Input: dimensioned drawing with shaded views. Units: mm. Origin: part minimum x, y, z. Round coordinates to 2 decimals unless told otherwise and drop trailing zeros. Loops run counter-clockwise (first coordinate to the right, second up) from the corner with the lowest first, then second, coordinate; pieces in that order, holes last. Notation, with made-up numbers: M -36,-1 L -26,-1 A12 cw -26,17 Z; hole C -35.75,64.5 d7. An arc over 180 degrees is marked long. Answer as a JSON object with one key per item and string values.
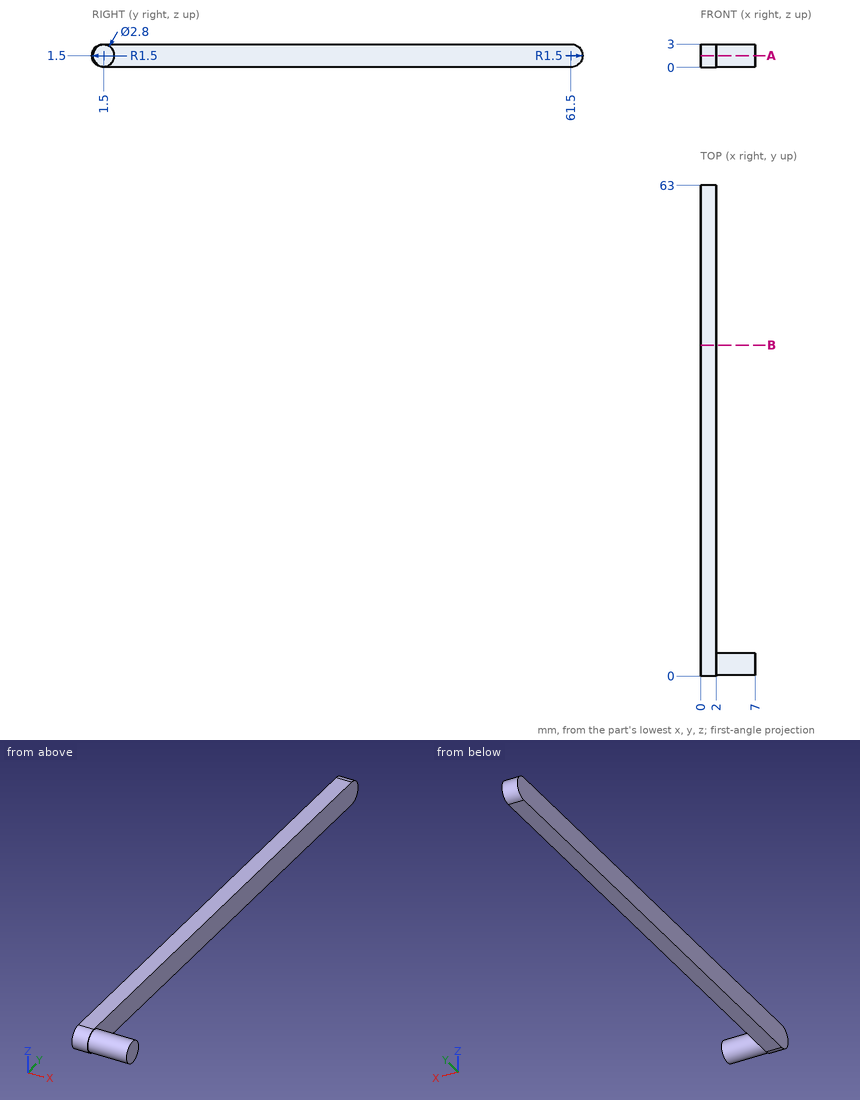
Item 1: Contact query for flat-ended pins moving along their axis: pin 1 Ø1 at (x, z) = (3, 2.5) entering from +Y; pin 2 Ø1.5 at (y, z) = (30, 2) entering from +X; pin 3 Ø1 at (x, z) = (5.5, 2.5) entering from -Y. Output: stop coordinate, or through.
Answer sheet:
{"pin 1": "stops at y = 2.81", "pin 2": "stops at x = 2", "pin 3": "stops at y = 0.19"}
Item 2: Section A-A on z = 1.5. Return the cut outline in (x, y), then the cut area to 3 significant figures.
Answer sheet:
{"outline": "M 0,0 L 2,0 L 2,0.1 L 7,0.1 L 7,2.9 L 2,2.9 L 2,63 L 0,63 Z", "area": "140 mm²"}
Item 3: Line query: probe 1 along X at (y, z) = (17.5, 1.6); probe 2 along Y at (x, z) = (3, 2.3); probe 3 along Y at (x, z) = (1.5, 1.8). Output: solid intervals per line, ascending. Write a range as from..to.
Answer sheet:
{"probe 1": "x = 0..2", "probe 2": "y = 0.35..2.65", "probe 3": "y = 0.03..62.97"}
Item 4: Section B-B on y = 42.5. Return the cut outline in (x, z), then the cut area to 3 significant figures.
Answer sheet:
{"outline": "M 0,0 L 2,0 L 2,3 L 0,3 Z", "area": "6.00 mm²"}
